```python
from build123d import *

# Parameters (mm, degrees)
F1_DEPTH  = 35
F2_W      = 6.8124607205
F2_H      = 15.0619698688
F3_DEPTH  = 70
F5_DEPTH  = 70
F6_W      = 3
F6_H      = 3
F7_DEPTH  = 10
F8_W      = 3
F8_H      = 2
F9_DEPTH  = 10
F11_DEPTH = 3


with BuildPart() as f1:
    # F0 (on Right) → F1 (new body, symmetric)
    with BuildSketch(Plane.YZ):
        Polygon((-20.4803533852, 0), (0, 0), (25.0509791076, 0), (25.0509791076, 27.6123592876), (-9.8410505696, 27.6123592876), align=None)
    extrude(amount=F1_DEPTH, both=True)

    # F2 (on face) → F3 (cut, through all)
    with BuildSketch(Plane.YZ.offset(35)):
        Polygon((7.0281750523, 27.6123592876), (1.9915826587, 27.6123592876), (0.1867247932, 12.7213389033), (1.6758268317, 12.5408531167), (0.7132359701, 4.5989755784), (2.6987053547, 4.358327863), (3.6612962162, 12.3002054013), (5.1503982547, 12.1197196148), align=None)
        Polygon((-13.6446588918, 4.256867985), (-11.2603206785, 23.9289040036), (-18.6083323532, 4.8584872735), align=None)
        with Locations((21.6447487473, 20.0813743531)):
            Rectangle(F2_W, F2_H)
    extrude(amount=-F3_DEPTH, mode=Mode.SUBTRACT)

    # F4 (on face) → F5 (cut, through all)
    with BuildSketch(Plane.YZ.offset(35)):
        Polygon((-11.2603206785, 23.9289040036), (-11.5959745991, 21.1595837877), (1.2094775837, 21.1595837877), (1.9915826587, 27.6123592876), (-9.8410505696, 27.6123592876), align=None)
    extrude(amount=-F5_DEPTH, mode=Mode.SUBTRACT)

    # F6 (on face) → F7 (join)
    with BuildSketch(Plane(origin=(0, 0.3109364051, 2.5653877984), x_dir=(1, 0, 0), z_dir=(0, 0.1203238577, 0.9927346923))):
        with Locations((11.5, -17.557729024)):
            Rectangle(F6_W, F6_H)
        with Locations((-11.5, -17.557729024)):
            Rectangle(F6_W, F6_H)
    extrude(amount=F7_DEPTH)

    # F8 (on face) → F9 (join)
    with BuildSketch(Plane.XY.offset(12.5503894187)):
        with Locations((33.5, 24.0509791076)):
            Rectangle(F8_W, F8_H)
        with Locations((-33.5, 24.0509791076)):
            Rectangle(F8_W, F8_H)
    extrude(amount=F9_DEPTH)

    # F10 (on face) → F11 (cut)
    with BuildSketch(Plane(origin=(0, 25.0509791076, 0), x_dir=(-1, 0, 0), z_dir=(0, 1, 0))):
        Polygon((13, 12.5503894187), (0, 12.5503894187), (-13, 12.5503894187), (-13, 2.5503894187), (13, 2.5503894187), align=None)
    extrude(amount=-F11_DEPTH, mode=Mode.SUBTRACT)


solid = f1.part
```
Input: part model. Units: mm. Frame: model coordinates. A direction names the side the tool comes from. Give positions to 0.01 mm unless a question says otherwise; leave off trailing zeros. Loops run counter-clockwise (first coordinate to the right, second up) from the corner with the lowest first, then second, coordinate; pieces in that order, holes last. Notation, with made-up numbers: (81.25, 77.25) -> (140.25, 77.25) arc R35 cw to (140.25, 112.25) -> close; hole circle Ø7 at (-25.5, -16). An arc over 180 degrees is marked (long way). Use a Markdown table: item, result.
Q1. Section query A-A, the plane z = 6.25. Return the cut outline in (x, y), plus the area to 3 significant figures.
Entries:
| item | result |
|---|---|
| outline | (-35, -13.4) -> (35, -13.4) -> (35, 0.91) -> (-35, 0.91) -> close; (-35, 2.93) -> (35, 2.93) -> (35, 25.05) -> (13, 25.05) -> (13, 22.05) -> (-13, 22.05) -> (-13, 25.05) -> (-35, 25.05) -> close; (-13, -18.44) -> (-10, -18.44) -> (-10, -15.42) -> (-13, -15.42) -> close; (10, -18.44) -> (13, -18.44) -> (13, -15.42) -> (10, -15.42) -> close |
| area | 2,490 mm² |
Q2. Section query B-B, the plane x = 22. Return the cut outline in (y, z), plus the area to 3 significant figures.
Entries:
| item | result |
|---|---|
| outline | (-20.48, 0) -> (25.05, 0) -> (25.05, 12.55) -> (18.24, 12.55) -> (18.24, 27.61) -> (7.03, 27.61) -> (5.15, 12.12) -> (3.66, 12.3) -> (2.7, 4.36) -> (0.71, 4.6) -> (1.68, 12.54) -> (0.19, 12.72) -> (1.21, 21.16) -> (-11.6, 21.16) -> (-13.64, 4.26) -> (-18.61, 4.86) -> close |
| area | 785 mm² |
Q3. Access query for faces 1 (the flat face through (35, 7, 11)), 2 (the flat face through (0.49, 0.705, 17)), 3 (the flat face through (-34, 24, 22.55)), 4 (the flat face through (0.49, 3.173, 8.274)), 5 (the flat face through (0, 2, 0)). Directions: +Z, -Z, +X, -X, +Y, -Y. A direction counts if a zero-diameter tool reaches every point of the face in a straight line with its end or side. Return the directions, or none.
Entries:
| item | result |
|---|---|
| face 1 | +Z, -Z, +X, +Y, -Y |
| face 2 | +X, -X |
| face 3 | +Z, +X, -X, +Y |
| face 4 | +Z, +X, -X |
| face 5 | -Z, +X, -X, +Y, -Y |
Q4. Section query C-C, the plane y = -9. Return the cut outline in (x, z), plus the area to 3 significant figures.
Entries:
| item | result |
|---|---|
| outline | (-35, 0) -> (35, 0) -> (35, 21.16) -> (-35, 21.16) -> close |
| area | 1,480 mm² |
Q5. Section query D-D, the plane z = 19.25. Return the cut outline in (x, y), plus the area to 3 significant figures.
Entries:
| item | result |
|---|---|
| outline | (-35, -11.83) -> (35, -11.83) -> (35, 0.98) -> (-35, 0.98) -> close; (-35, 6.01) -> (35, 6.01) -> (35, 18.24) -> (-35, 18.24) -> close; (-35, 23.05) -> (-32, 23.05) -> (-32, 25.05) -> (-35, 25.05) -> close; (32, 23.05) -> (35, 23.05) -> (35, 25.05) -> (32, 25.05) -> close |
| area | 1,760 mm² |
Q6. Pull-direction query (X, two-part tool) for faces 6 (the flat face through (0, 25.051, 1)), 7 (the flat face through (-10, -17, 10)), 8 (the flat face through (-35, 7, 11)); classes: pulls with the +X half, pulls with the -X half, needs draft (parallel to the pull), parting line crosses it, or undercut.
Entries:
| item | result |
|---|---|
| face 6 | needs draft |
| face 7 | undercut |
| face 8 | pulls with the -X half |
Q7. First-contact query: P1, Ø8, axis at x = -27, y = 19, coming from the -Z side; P2, Ø1.3, axis at y = -16.5, z = 7.5, coming from the +X side; P3, Ø11, axis at x = -5, z = 9, coming from the +Y side; P4, Ø0.6, axis at x = 33, y = 24, coming from the +Z side. Flat tips, straight axial feed; report the tip coordinate or a pass-through.
Entries:
| item | result |
|---|---|
| P1 | stops at z = 0 |
| P2 | stops at x = 13 |
| P3 | stops at y = 22.05 |
| P4 | stops at z = 22.55 |
Q8. Ray query, probe 1 along X at (y, z) = (-16, 12.75); probe 2 along X at (y, z) = (23, 9.25); probe 3 along Z at (x, y) = (16, -5). Return the intervals inside material, ascending. Write a range as from..to.
Entries:
| item | result |
|---|---|
| probe 1 | x = -13..-10, 10..13 |
| probe 2 | x = -35..-13, 13..35 |
| probe 3 | z = 0..21.16 |
